Check sheet for the modelled part. Datum: model origin and axes. Units: mm. Face numbers are marked on the shaded views. A direction names the side the tool comes from. Give positions to 0.01 mm unless a question says otherwise; leave off trailing zeros. Order: outer loops, then holes, each group sorted by start corner. A loop starts at its lowest first (then second) coordinate and runs counter-clockwise, first axis right, second up.
Item 1: Sectioned sample at D-D on x = 19.5. Record the boundary of the cut face in (y, z), and give its area (3 significant figures).
Item 2: Release check for a two-part mould opening along Z. For the marked faces 1, 2 and 3 record: released by +Z, released by -Z, zero draft, split by the parting line, or undercut.
Item 3: Sectioned sample at C-C on y = 17. Record the boundary of the cut face in (x, z), and give its area (3 significant figures).
Item 4: Sectioned sample at B-B on z = 0. Record the boundary of the cut face in (x, y), and give its area (3 significant figures).
Item 5: Gauge pin test, flat ends, axial feed: P1, Ø19.5, axis at x = 0, z = 67.5, coming from the -Y side; P2, Ø24, axis at x = -58.46, z = -33.75, coming from the +Y side; P3, Ø10, axis at x = -25.5, y = 14, coming from the +Z side; P4, Ø8, axis at x = -32, z = 41.5, coming from the +Y side. Record the tip position at first contact, or that the pin passes through.
Item 6: Access from +Z, -Z, +X, -X, +Y, -Y to the whole of each face (thin tool, end or side, straight path). Record for the marked faces 4 and 5.
Item 7: Sectioned sample at A-A on x = 0. Record the boundary of the cut face in (y, z), and give its area (3 significant figures).
Item 8: Material ranges on line 1 along X through (y, z) = (1.3, 33.75); line 2 along Z through (x, y) = (-1.5, 2.5); line 3 along Z through (x, y) = (-1, 5.25), recorded low to high.
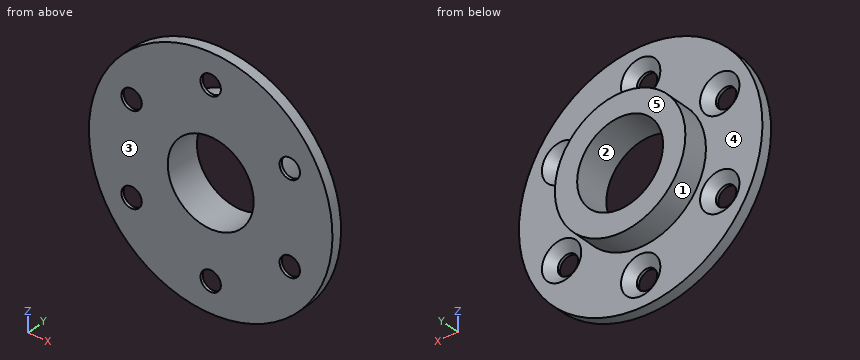
from build123d import *

# Parameters (mm, degrees)
SKETCH5_R           = 90
BOSS_EXTRUDE1_DEPTH = 8
SKETCH6_R           = 48.25
SKETCH6_R_2         = 31.75
EXTRUDE_THIN1_DEPTH = 19
CIRPATTERN1_COUNT   = 6
SKETCH13_W          = 31.75
SKETCH13_H          = 30.969260742


with BuildPart() as part:
    # Sketch5 → Boss-Extrude1 (new body)
    with BuildSketch(Plane(origin=(0, 0, 0), x_dir=(1, 0, 0), z_dir=(0, 1, 0))):
        with Locations(Location((0, 0, 0), (0, 0, 270))):
            Circle(SKETCH5_R)
    extrude(amount=BOSS_EXTRUDE1_DEPTH)

    # Sketch6 → Extrude-Thin1 (add)
    with BuildSketch(Plane(origin=(0, 8, 0), x_dir=(1, 0, 0), z_dir=(0, 1, 0))):
        Circle(SKETCH6_R)
        Circle(SKETCH6_R_2, mode=Mode.SUBTRACT)
    extrude(amount=EXTRUDE_THIN1_DEPTH)

    # Sketch10 → CSK for 9/16 Flat Head Machine Screw (100)1 (revolve, cut)
    with BuildSketch(Plane(origin=(0, 8, -67.5), x_dir=(0, 0, 1), z_dir=(1, 0, 0))):
        Polygon((0, 0), (0, 8), (7.53999, 8), (7.53999, 5.874964459), (14.5415, 0), align=None)
    csk_for_9_16_flat_head_machine_screw_10 = revolve(axis=Axis((0, 14.35, -67.5), (0, -1, 0)), mode=Mode.SUBTRACT)

    # CirPattern1: CSK for 9/16 Flat Head Machine Screw (100)1 ×6 about axis
    cirpattern1_axis = Axis((0, 0, 0), (0, 1, 0))
    for i in range(1, CIRPATTERN1_COUNT):
        add(csk_for_9_16_flat_head_machine_screw_10.rotate(cirpattern1_axis, i * 360 / CIRPATTERN1_COUNT), mode=Mode.SUBTRACT)

    # Sketch13 → Cut-Revolve1 (revolve, cut)
    with BuildSketch(Plane.XY, mode=Mode.PRIVATE) as cut_revolve1_sk:
        with Locations((-15.875, 11.515369629)):
            Rectangle(SKETCH13_W, SKETCH13_H)
    revolve(cut_revolve1_sk.sketch.rotate(Axis((0, 27, 0), (0, -1, 0)), 180), axis=Axis((0, 27, 0), (0, -1, 0)), mode=Mode.SUBTRACT)


solid = part.part
Report:
1. outline: (0, -87.86) - (8, -87.86) - (8, -44.13) - (27, -44.13) - (27, -25.06) - (0, -25.06) - close; (0, 25.06) - (27, 25.06) - (27, 44.13) - (8, 44.13) - (8, 87.86) - (0, 87.86) - close
1. area: 1,730 mm2
2. face 1: split by the parting line
2. face 2: undercut
2. face 3: zero draft
3. outline: circle Ø96.5 at (0, 0); hole circle Ø63.5 at (0, 0)
3. area: 4,150 mm2
4. outline: (-90, 0) - (-31.75, 0) - (-31.75, 27) - (-48.25, 27) - (-48.25, 8) - (-90, 8) - close; (31.75, 0) - (90, 0) - (90, 8) - (48.25, 8) - (48.25, 27) - (31.75, 27) - close
4. area: 1,560 mm2
5. P1: stops at y = 0
5. P2: stops at y = 5.87
5. P3: stops at z = 43.68
5. P4: stops at y = 8
6. face 4: +Y
6. face 5: +Z, -Z, +X, -X, +Y
7. outline: (0, -90) - (8, -90) - (8, -82.04) - (2.13, -75.04) - (0, -75.04) - close; (0, -59.96) - (2.13, -59.96) - (8, -52.96) - (8, -48.25) - (27, -48.25) - (27, -31.75) - (0, -31.75) - close; (0, 31.75) - (27, 31.75) - (27, 48.25) - (8, 48.25) - (8, 52.96) - (2.13, 59.96) - (0, 59.96) - close; (0, 75.04) - (2.13, 75.04) - (8, 82.04) - (8, 90) - (0, 90) - close
7. area: 1,240 mm2
8. line 1: x = -83.43 to -66, -50.92 to 50.92, 66 to 83.43
8. line 2: z = -89.99 to -75.34, -59.66 to -31.71, 31.71 to 59.66, 75.34 to 89.99
8. line 3: z = -89.99 to -78.72, -56.28 to -31.73, 31.73 to 56.28, 78.72 to 89.99
